from build123d import *

# Parameters (mm, degrees)
SKETCH1_R           = 2.035533906
SKETCH1_R_2         = 1.5
BOSS_EXTRUDE1_DEPTH = 1
SKETCH1_3_W         = 20
SKETCH1_3_H         = 20
BOSS_EXTRUDE2_DEPTH = 1


with BuildPart() as part:
    # Sketch1 → Boss-Extrude1 (new body)
    with BuildSketch(Plane(origin=(0, 0, 0), x_dir=(1, 0, 0), z_dir=(0, 1, 0))):
        Polygon((1, 7.499999998), (1, 12.5), (1, 17.5), (0, 17.5), (0, 0), (20, 0), (20, 20), (2.5, 20), (2.5, 19), (7.5, 19), (12.500000017, 19), (17.5, 19), (19, 19), (19, 17.5), (19, 12.5), (19, 7.5), (19, 2.5), (19, 1), (17.5, 1), (12.49999999, 1), (7.5, 1), (2.5, 1), (1, 1), (1, 2.5), align=None)
        with Locations((5, 5)):
            Circle(SKETCH1_R)
        with Locations((5, 5)):
            Circle(SKETCH1_R_2, mode=Mode.SUBTRACT)
        with Locations((5, 10)):
            Circle(SKETCH1_R)
        with Locations((5, 10)):
            Circle(SKETCH1_R_2, mode=Mode.SUBTRACT)
        with BuildLine():
            ThreePointArc((3.560660176, 16.439339833), (2.964466094, 15.000000004), (3.560660171, 13.560660172))
            Line((3.560660172, 13.560660172), (3.939339828, 13.939339828))
            ThreePointArc((3.939339828, 13.939339828), (3.939339828, 16.060660172), (6.060660172, 16.060660172))
            Line((6.060660172, 16.060660172), (6.439339828, 16.439339828))
            ThreePointArc((6.439339828, 16.439339829), (5.000000003, 17.035533906), (3.560660176, 16.439339833))
        make_face()
        with BuildLine():
            Line((3.939339828, 13.939339828), (3.560660172, 13.560660172))
            ThreePointArc((3.560660171, 13.560660172), (5, 12.964466094), (6.439339828, 13.560660172))
            ThreePointArc((6.439339828, 13.560660172), (6.880588113, 14.221034898), (7.035533906, 15))
            ThreePointArc((7.035533906, 15), (6.880588113, 15.778965102), (6.439339828, 16.439339829))
            Line((6.439339828, 16.439339828), (6.060660172, 16.060660172))
            ThreePointArc((6.060660172, 16.060660172), (6.385819299, 15.574025149), (6.5, 15))
            ThreePointArc((6.5, 15), (5.574025149, 13.614180701), (3.939339828, 13.939339828))
        make_face()
        with Locations((10, 5)):
            Circle(SKETCH1_R)
        with Locations((10, 5)):
            Circle(SKETCH1_R_2, mode=Mode.SUBTRACT)
        with Locations((15, 5)):
            Circle(SKETCH1_R)
        with Locations((15, 5)):
            Circle(SKETCH1_R_2, mode=Mode.SUBTRACT)
        with Locations((15, 15)):
            Circle(SKETCH1_R)
        with Locations((15, 15)):
            Circle(SKETCH1_R_2, mode=Mode.SUBTRACT)
        with Locations((15, 10)):
            Circle(SKETCH1_R)
        with Locations((15, 10)):
            Circle(SKETCH1_R_2, mode=Mode.SUBTRACT)
        with Locations((10, 10)):
            Circle(SKETCH1_R)
        with Locations((10, 10)):
            Circle(SKETCH1_R_2, mode=Mode.SUBTRACT)
        with Locations((10, 15)):
            Circle(SKETCH1_R)
        with Locations((10, 15)):
            Circle(SKETCH1_R_2, mode=Mode.SUBTRACT)
        Polygon((0, 17.5), (1, 17.5), (1, 19), (2.5, 19), (2.5, 20), (0, 20), align=None)
    extrude(amount=-BOSS_EXTRUDE1_DEPTH)

    # Sketch1_3 → Boss-Extrude2 (add)
    with BuildSketch(Plane(origin=(0, 0, 0), x_dir=(1, 0, 0), z_dir=(0, 1, 0))):
        with Locations((10, 10)):
            Rectangle(SKETCH1_3_W, SKETCH1_3_H)
    extrude(amount=BOSS_EXTRUDE2_DEPTH)


solid = part.part
Work out the finished part from the listing and answer in its coordinate system (mm). A direction names the side the tool comes from. Coordinates: 2 decimals unless noted, no trailing zeros. Loops run counter-clockwise (first coordinate to the right, second up) from the corner with the lowest first, then second, coordinate; pieces in that order, holes last. Notation, with made-up numbers: M 69,38 L 74,38 A30 ccw 74,65 Z; hole C -35,-31 d9. An arc over 180 degrees is marked long. Answer in a Markdown table with one row per item. Add a question column.
1. The mould has two halves that part along X. Classify faces 1 (the flat face through (15, 0, -15)), 2 (the flat face through (10, 1, -10)), 3 (the flat face through (20, 0, -10)): pulls with the +X half, pulls with the -X half, needs draft (parallel to the pull), parting line crosses it, or undercut.
2. Find section B-B, the plane x = 2.5. Write down the section's boundary in (y, z).
3. Find section A-A, the plane z = -1.5. Write down the section's boundary in (x, y), then the cut area to 3 significant figures.
4. Consider L1, parallel to X at y = -0.1, z = -2; L2, parallel to Y at x = 17, z = -2.25; L3, parallel to X at y = -0.45, z = -8.25. Determine where each line is inside the solid, lowest interval first.
5. A flat-ended cylindrical pin translates along its axis: P1, Ø2.5, axis at x = 15, z = -15, coming from the -Y side. Find the tip coordinate at first contact, or state that the pin passes through.
6. A tool of negligible diameter and unlimited length cuts with its end or side. For faces 4 (the flat face through (10.1, -0.5, -1)), 5 (the flat face through (10, 0, -20)), from which of +Z, -Z, +X, -X, +Y, -Y can it reach the whole face along a straight path? Write none if from no direction.
Reported:
| question | item | result |
|---|---|---|
| 1 | face 1 | undercut |
| 1 | face 2 | needs draft |
| 1 | face 3 | pulls with the +X half |
| 2 | outline | M -1,-20 L 1,-20 L 1,0 L -1,0 L -1,-1 L 0,-1 L 0,-19 L -1,-19 Z |
| 3 | outline | M 0,-1 L 1,-1 L 1,0 L 19,0 L 19,-1 L 20,-1 L 20,1 L 0,1 Z |
| 3 | area | 22.0 mm^2 |
| 4 | L1 | x = 0 to 1, 19 to 20 |
| 4 | L2 | y = 0 to 1 |
| 4 | L3 | x = 0 to 1, 3.96 to 6.04, 8.96 to 11.04, 13.96 to 16.04, 19 to 20 |
| 5 | P1 | stops at y = 0 |
| 6 | face 4 | -Y |
| 6 | face 5 | -Z, +X, -X, +Y, -Y |
